Source: CAD feature listing. Evaluate the final solid. Frame: model axes, mm. Face numbers are marked on the shaded views. A direction names the side the tool comes from. Coordinates: 2 decimals unless noted, no trailing zeros. Write each loop counter-clockwise with the first axis right and the second up, starting at its lowest first coordinate (ties: lowest second). Pieces come first, ordered by that corner, then holes. Notation, with made-up numbers: M -26.75,37 L 29.25,37 A31 cw 29.25,72 Z; hole C 82,-24 d7. An arc over 180 degrees is marked long. One line per item, written item: value. Start each with the question number.
Item 1: Ray query, L1, parallel to X at y = 22, z = -7.25; L2, parallel to X at y = 10, z = -7.75; L3, parallel to Y at x = 25, z = 0.25. Return the intervals inside material, ascending. Write a range as from..to.
Item 2: Cut plane B-B, the plane z = 1.5. Output: boundary loops of the cut face in (x, y).
Item 3: Pin query (flat end, axial travel): P1, Ø3, axis at x = 40.77, y = 22, coming from the +Z side; P2, Ø8, axis at x = -17, y = 22.5, coming from the +Z side; P3, Ø4.5, axis at x = 50, y = 22, coming from the -Z side. Return the tip coordinate at first contact, or that it passes through.
Item 4: Cut plane D-D, the plane y = 15. Output: boundary loops of the cut face in (x, z) (1 decimal).
Item 5: Cut plane A-A, the plane y = -6. Output: boundary loops of the cut face in (x, z) (1 decimal).
Item 6: Set-up query: the marked faces 1, 2 and 3. Return all of +Z, -Z, +X, -X, +Y, -Y with unobstructed straight access to the full face (end or side cutting, diameter ignored); none if empty.
Item 7: Cut plane C-C, the plane x = -1. Output: boundary loops of the cut face in (y, z).
Item 8: Mould query, pull axis Y, two halves, no side actions, for the marked faces 4, 5, 6 and 7. Classes: released by +Y, released by -Y, zero draft, split by the parting line, or undercut.
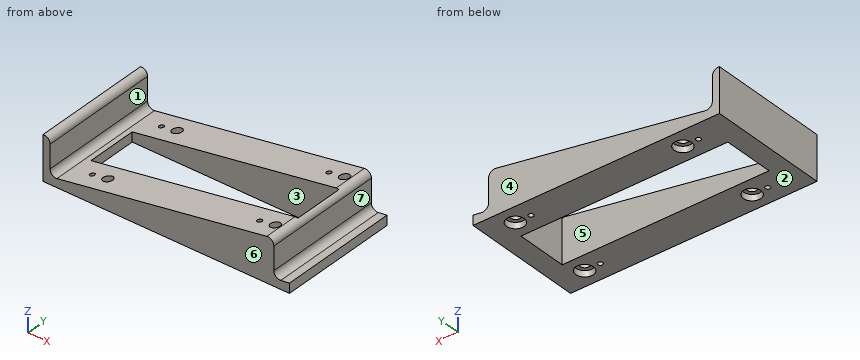
```python
from build123d import *

# Parameters (mm, degrees)
F1_DEPTH = 31
F3_W     = 106.2213294208
F3_H     = 13.1045691669
F4_DEPTH = 25
F5_R     = 1.25
F5_R_2   = 2.5
F6_DEPTH = 15
F7_START = -8
F5_R_3   = 4.5
F7_DEPTH = 4


with BuildPart() as f1:
    # F0 (on Front) → F1 (new body)
    with BuildSketch(Plane.XZ):
        with BuildLine():
            Line((-59.654000323, -3.5138892937), (-59.654000323, 8.3879307063))
            ThreePointArc((-59.654000323, 8.3879307063), (-60.7190612433, 10.8045648955), (-63.2520458808, 11.5518696492))
            Line((-63.2520458808, 11.5518696492), (-63.2789134979, -11.1016744181))
            Line((-63.2789134979, -11.1016744181), (63.284156729, -11.1016744181))
            Line((63.284156729, -11.1016744181), (63.284156729, -6.1260935991))
            Line((63.284156729, -6.1260935991), (58.8121598262, -6.7381653853))
            ThreePointArc((58.8121598262, -6.7381653853), (56.307949738, -5.9657950954), (55.2598693261, -3.5638892937))
            Line((55.2598693261, -3.5638892937), (55.2598693261, 8.3326508177))
            ThreePointArc((55.2598693261, 8.3326508177), (54.1975321527, 10.7659194445), (51.649858136, 11.5133909047))
            Line((51.649858136, 11.5133909047), (-56.1369696956, -6.6881653853))
            ThreePointArc((-56.1369696956, -6.6881653853), (-58.6174350193, -5.900932648), (-59.654000323, -3.5138892937))
        make_face()
    extrude(amount=F1_DEPTH)

    # F2: F1 across plane


with BuildPart() as f1_1:
    add(f1.part)
    add(f1.part.mirror(Plane.XZ))

    # F3 (on Top) → F4 (cut, symmetric)
    with BuildSketch(Plane.XY):
        with Locations((0.0008549541, -6.5522845834)):
            Rectangle(F3_W, F3_H)
        with Locations((0.0008549541, 6.5522845834)):
            Rectangle(F3_W, F3_H)
    extrude(amount=F4_DEPTH, both=True, mode=Mode.SUBTRACT)

    # F5 (on Top) → F6 (cut, symmetric)
    with BuildSketch(Plane.XY):
        with Locations((40.7651439339, -22)):
            Circle(F5_R)
        with Locations((-45.2348560661, -21.9999999583)):
            Circle(F5_R)
        with Locations((-45.23294, 22)):
            Circle(F5_R)
        with Locations((40.76706, 22)):
            Circle(F5_R)
        with Locations((-37.23294, 22)):
            Circle(F5_R_2)
        with Locations((-37.2348560737, -22.0003483339)):
            Circle(F5_R_2)
        with Locations((48.7651439263, -22.0003483756)):
            Circle(F5_R_2)
        with Locations((48.76706, 22)):
            Circle(F5_R_2)
    extrude(amount=F6_DEPTH, both=True, mode=Mode.SUBTRACT)

    # F5 (on Top) → F7 (cut)
    with BuildSketch(Plane.XY.offset(F7_START)):
        with Locations((-37.23294, 22)):
            Circle(F5_R_3)
        with Locations((-37.23294, 22)):
            Circle(F5_R_2, mode=Mode.SUBTRACT)
        with Locations((-37.2348560737, -22.0003483339)):
            Circle(F5_R_3)
        with Locations((-37.2348560737, -22.0003483339)):
            Circle(F5_R_2, mode=Mode.SUBTRACT)
        with Locations((48.76706, 22)):
            Circle(F5_R_3)
        with Locations((48.76706, 22)):
            Circle(F5_R_2, mode=Mode.SUBTRACT)
        with Locations((48.7651439263, -22.0003483756)):
            Circle(F5_R_3)
        with Locations((48.7651439263, -22.0003483756)):
            Circle(F5_R_2, mode=Mode.SUBTRACT)
    extrude(amount=-F7_DEPTH, mode=Mode.SUBTRACT)


solid = f1_1.part
```
From the geometry:
1. L1: x = -63.27..-46.48, -43.98..-39.73, -34.73..39.52, 42.02..46.27, 51.27..63.28
1. L2: x = -63.27..-53.11, 53.11..63.28
1. L3: y = -31..-13.1, 13.1..31
2. outline: M -63.26,-31 L -59.65,-31 L -59.65,31 L -63.26,31 Z; M -7.65,-31 L 55.26,-31 L 55.26,31 L -7.65,31 L -7.65,13.1 L 53.11,13.1 L 53.11,-13.1 L -7.65,-13.1 Z; hole C 40.77,-22 d2.5; hole C 40.77,22 d2.5; hole C 48.77,-22 d5; hole C 48.77,22 d5
3. P1: stops at z = 9.93
3. P2: stops at z = 0.6
3. P3: stops at z = -8
4. outline: M -63.3,-11.1 L 63.3,-11.1 L 63.3,-6.1 L 58.8,-6.7 A3.1 cw 55.3,-3.6 L 55.3,8.3 A3.1 ccw 51.6,11.5 L -56.1,-6.7 A3.1 cw -59.7,-3.5 L -59.7,8.4 A3.1 ccw -63.3,11.6 Z
5. outline: M -63.3,-11.1 L -53.1,-11.1 L -53.1,-6.2 L -56.1,-6.7 A3.1 cw -59.7,-3.5 L -59.7,8.4 A3.1 ccw -63.3,11.6 Z; M 53.1,-11.1 L 63.3,-11.1 L 63.3,-6.1 L 58.8,-6.7 A3.1 cw 55.3,-3.6 L 55.3,8.3 A3.1 ccw 53.1,11.4 Z
6. face 1: +Z, +Y, -Y
6. face 2: -Z, +X, -X, +Y, -Y
6. face 3: +Z, -Z
7. outline: M -31,-11.1 L -13.1,-11.1 L -13.1,2.62 L -31,2.62 Z; M 13.1,-11.1 L 31,-11.1 L 31,2.62 L 13.1,2.62 Z
8. face 4: released by +Y
8. face 5: undercut
8. face 6: released by -Y
8. face 7: zero draft
